Source: three-view drawing plus pictorial views. Frame: mm from the lowest corner of the part. A direction names the side the tool comes from. Give positions to 0.01 mm unless a question says otherwise; leave off trailing zeros. Order: outer loops, then holes, each group sorted by start corner. A loop starts at its lowest first (then second) coordinate and runs counter-clockwise, first axis right, second up.
1) First-contact query: P1, Ø1.5, axis at x = 12.5, z = 11.5, coming from the -Y side; P2, Ø2.5, axis at x = 51.19, y = 25.31, coming from the +Z side; P3, Ø3, axis at x = 28, y = 25.5, coming from the +Z side. Flat tips, straight axial feed; report the tip coordinate or a pass-through.
2) Section D-D, the plane x = 17. Return loops of the section in (y, z), plus the area to 3 significant figures.
3) Section B-B, the plane z = 32.5. Return loops of the section in (x, y).
4) Section A-A, the plane x = 27.5. Return loops of the section in (y, z).
5) Material intervals for line 1 (Y direction, x = 3, z = 52); line 2 (Z direction, x = 34, y = 1.5); line 3 (Z direction, x = 27.5, y = 12), sorted ascending.
6) Section C-C, the plane y = 10.75. Return loops of the section in (x, z).
7) Access query for the marked faces 5, 6 and 7. Directions: +Z, -Z, +X, -X, +Y, -Y. A direction counts if a zero-diameter tool reaches every point of the face in a straight line with its end or side. Return the directions, or none.
8) Draft query along X for the marked faces 1, 2, 3 and 4. Return one class per face: released by +X, released by -X, zero draft, split by the parting line, or undercut.
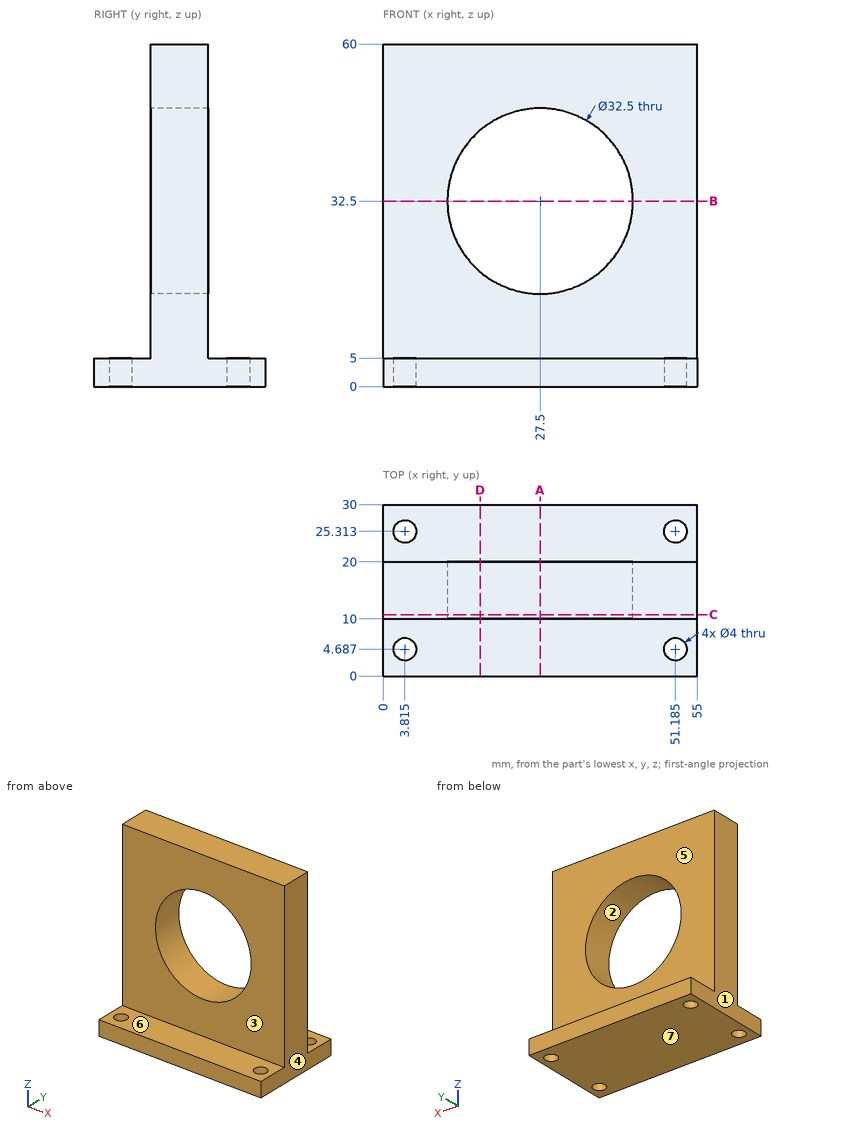
From the geometry:
1. P1: stops at y = 10
1. P2: passes through
1. P3: stops at z = 5
2. outline: (0, 0) - (30, 0) - (30, 5) - (20, 5) - (20, 20.1) - (10, 20.1) - (10, 5) - (0, 5) - close; (10, 44.9) - (20, 44.9) - (20, 60) - (10, 60) - close
2. area: 452 mm2
3. outline: (0, 10) - (11.25, 10) - (11.25, 20) - (0, 20) - close; (43.75, 10) - (55, 10) - (55, 20) - (43.75, 20) - close
4. outline: (0, 0) - (30, 0) - (30, 5) - (20, 5) - (20, 16.25) - (10, 16.25) - (10, 5) - (0, 5) - close; (10, 48.75) - (20, 48.75) - (20, 60) - (10, 60) - close
5. line 1: y = 10 to 20
5. line 2: z = 0 to 5
5. line 3: z = 0 to 16.25, 48.75 to 60
6. outline: (0, 0) - (55, 0) - (55, 60) - (0, 60) - close; hole circle Ø32.5 at (27.5, 32.5)
7. face 5: +Z, +X, -X, +Y
7. face 6: +Z, +X, -X, -Y
7. face 7: -Z, +X, -X, +Y, -Y
8. face 1: released by -X
8. face 2: undercut
8. face 3: zero draft
8. face 4: released by +X
